Check sheet for the modelled part. Datum: model origin and axes. Units: mm. Face numbers are marked on the shaded views. A direction names the side the tool comes from. Give positions to 0.01 mm unless a question says otherwise; leave off trailing zeros. Write each loop counter-clockwise with the first axis right and the second up, starting at its lowest first coordinate (ties: lowest second). Pieces come first, ordered by that corner, then holes. Notation, with made-up numbers: (-20, 89) -> (4, 89) arc R20 cw to (4, 107) -> close; hole circle Ø10 at (-5, 18). An arc over 180 degrees is marked (long way). Write each question's results on one line, items separated by ' | '. Start each with the question number.
```python
from build123d import *

# Parameters (mm, degrees)
CYLINDER051_R             = 1.6
CYLINDER051_DEPTH         = 28
CYLINDER051_ROLL_ANGLE    = 90
CYLINDER050_R             = 1.6
CYLINDER050_DEPTH         = 28
CYLINDER050_ROLL_ANGLE    = 90
CYLINDER049_R             = 1.6
CYLINDER049_DEPTH         = 28
CYLINDER049_ROLL_ANGLE    = 90
CYLINDER048_R             = 1.6
CYLINDER048_DEPTH         = 28
CYLINDER048_ROLL_ANGLE    = 90
CYLINDER044_R             = 1.6
CYLINDER044_DEPTH         = 28
CYLINDER044_ROLL_ANGLE    = 90
CYLINDER043_R             = 1.6
CYLINDER043_DEPTH         = 28
CYLINDER043_ROLL_ANGLE    = 90
CYLINDER042_R             = 1.6
CYLINDER042_DEPTH         = 28
CYLINDER042_ROLL_ANGLE    = 90
CYLINDER041_R             = 1.6
CYLINDER041_DEPTH         = 28
CYLINDER041_ROLL_ANGLE    = 90
CYLINDER047_R             = 0.85
CYLINDER047_DEPTH         = 10
CYLINDER046_R             = 0.85
CYLINDER046_DEPTH         = 10
FUSION078_PLACEMENT_ANGLE = 90
BOX025_W                  = 22
BOX025_H                  = 4
BOX025_DEPTH              = 5
CYLINDER045_R             = 3.25
CYLINDER045_DEPTH         = 10
CYLINDER045_PITCH_ANGLE   = 90
BOX024_W                  = 55
BOX024_H                  = 31
BOX024_DEPTH              = 13
BOX021_W                  = 61
BOX021_H                  = 34
BOX021_DEPTH              = 13
BOX023_W                  = 12
BOX023_H                  = 3
BOX023_DEPTH              = 13
BOX022_W                  = 12
BOX022_H                  = 3
BOX022_DEPTH              = 13


with BuildPart() as cylinder067:
    # Cylinder051 → Cylinder051 (new body)
    with BuildSketch(Plane.XY):
        Circle(CYLINDER051_R)
    extrude(amount=CYLINDER051_DEPTH)


with BuildPart() as cylinder067_1:
    # Cylinder051 roll: moved
    add(cylinder067.part.rotate(Axis((0, 0, 0), (1, 0, 0)), CYLINDER051_ROLL_ANGLE))


with BuildPart() as cylinder067_2:
    # Cylinder051 placement: moved
    add(cylinder067_1.part.moved(Location((-23, 20, 36))))


with BuildPart() as fusion085:
    # Cylinder050 → Cylinder050 (new body)
    with BuildSketch(Plane.XY):
        Circle(CYLINDER050_R)
    extrude(amount=CYLINDER050_DEPTH)


with BuildPart() as fusion085_1:
    # Cylinder050 roll: moved
    add(fusion085.part.rotate(Axis((0, 0, 0), (1, 0, 0)), CYLINDER050_ROLL_ANGLE))


with BuildPart() as fusion085_2:
    # Cylinder050 placement: moved
    add(fusion085_1.part.moved(Location((-23, 20, 29))))

    # Fusion085: union Cylinder067
    add(cylinder067_2.part)


with BuildPart() as fusion085_3:
    # Fusion085 placement: moved
    add(fusion085_2.part.moved(Location((-1, 0, 0))))


with BuildPart() as cylinder063:
    # Cylinder049 → Cylinder049 (new body)
    with BuildSketch(Plane.XY):
        Circle(CYLINDER049_R)
    extrude(amount=CYLINDER049_DEPTH)


with BuildPart() as cylinder063_1:
    # Cylinder049 roll: moved
    add(cylinder063.part.rotate(Axis((0, 0, 0), (1, 0, 0)), CYLINDER049_ROLL_ANGLE))


with BuildPart() as cylinder063_2:
    # Cylinder049 placement: moved
    add(cylinder063_1.part.moved(Location((-23, 20, 36))))


with BuildPart() as fusion084:
    # Cylinder048 → Cylinder048 (new body)
    with BuildSketch(Plane.XY):
        Circle(CYLINDER048_R)
    extrude(amount=CYLINDER048_DEPTH)


with BuildPart() as fusion084_1:
    # Cylinder048 roll: moved
    add(fusion084.part.rotate(Axis((0, 0, 0), (1, 0, 0)), CYLINDER048_ROLL_ANGLE))


with BuildPart() as fusion084_2:
    # Cylinder048 placement: moved
    add(fusion084_1.part.moved(Location((-23, 20, 29))))

    # Fusion084: union Cylinder063
    add(cylinder063_2.part)


with BuildPart() as fusion084_3:
    # Fusion084 placement: moved
    add(fusion084_2.part.moved(Location((1, 0, 0))))


with BuildPart() as cylinder054:
    # Cylinder044 → Cylinder044 (new body)
    with BuildSketch(Plane.XY):
        Circle(CYLINDER044_R)
    extrude(amount=CYLINDER044_DEPTH)


with BuildPart() as cylinder054_1:
    # Cylinder044 roll: moved
    add(cylinder054.part.rotate(Axis((0, 0, 0), (1, 0, 0)), CYLINDER044_ROLL_ANGLE))


with BuildPart() as cylinder054_2:
    # Cylinder044 placement: moved
    add(cylinder054_1.part.moved(Location((-23, 20, 36))))


with BuildPart() as fusion080:
    # Cylinder043 → Cylinder043 (new body)
    with BuildSketch(Plane.XY):
        Circle(CYLINDER043_R)
    extrude(amount=CYLINDER043_DEPTH)


with BuildPart() as fusion080_1:
    # Cylinder043 roll: moved
    add(fusion080.part.rotate(Axis((0, 0, 0), (1, 0, 0)), CYLINDER043_ROLL_ANGLE))


with BuildPart() as fusion080_2:
    # Cylinder043 placement: moved
    add(fusion080_1.part.moved(Location((-23, 20, 29))))

    # Fusion080: union Cylinder054
    add(cylinder054_2.part)


with BuildPart() as cylinder052:
    # Cylinder042 → Cylinder042 (new body)
    with BuildSketch(Plane.XY):
        Circle(CYLINDER042_R)
    extrude(amount=CYLINDER042_DEPTH)


with BuildPart() as cylinder052_1:
    # Cylinder042 roll: moved
    add(cylinder052.part.rotate(Axis((0, 0, 0), (1, 0, 0)), CYLINDER042_ROLL_ANGLE))


with BuildPart() as cylinder052_2:
    # Cylinder042 placement: moved
    add(cylinder052_1.part.moved(Location((54, 20, 36))))


with BuildPart() as fusion081:
    # Cylinder041 → Cylinder041 (new body)
    with BuildSketch(Plane.XY):
        Circle(CYLINDER041_R)
    extrude(amount=CYLINDER041_DEPTH)


with BuildPart() as fusion081_1:
    # Cylinder041 roll: moved
    add(fusion081.part.rotate(Axis((0, 0, 0), (1, 0, 0)), CYLINDER041_ROLL_ANGLE))


with BuildPart() as fusion081_2:
    # Cylinder041 placement: moved
    add(fusion081_1.part.moved(Location((54, 20, 29))))

    # Fusion081: union Cylinder052
    add(cylinder052_2.part)


with BuildPart() as cylinder059:
    # Cylinder047 → Cylinder047 (new body)
    with BuildSketch(Plane(origin=(10.5, -9, 0), x_dir=(1, 0, 0), z_dir=(0, 0, 1))):
        Circle(CYLINDER047_R)
    extrude(amount=CYLINDER047_DEPTH)


with BuildPart() as fusion078:
    # Cylinder046 → Cylinder046 (new body)
    with BuildSketch(Plane(origin=(10.5, 9, 0), x_dir=(1, 0, 0), z_dir=(0, 0, 1))):
        Circle(CYLINDER046_R)
    extrude(amount=CYLINDER046_DEPTH)

    # Fusion078: union Cylinder059
    add(cylinder059.part)


with BuildPart() as fusion078_1:
    # Fusion078 placement: moved
    add(fusion078.part.moved(Location((14.5, -39, 31))).rotate(Axis((14.5, -39, 31), (0, 0, 1)), FUSION078_PLACEMENT_ANGLE))


with BuildPart() as cut039:
    # Box025 → Box025 (new body)
    with BuildSketch(Plane(origin=(3.5, -31, 34), x_dir=(1, 0, 0), z_dir=(0, 0, 1))):
        with Locations((11, 2)):
            Rectangle(BOX025_W, BOX025_H)
    extrude(amount=BOX025_DEPTH)

    # Cut039: cut Fusion078
    add(fusion078_1.part, mode=Mode.SUBTRACT)


with BuildPart() as cylinder055:
    # Cylinder045 → Cylinder045 (new body)
    with BuildSketch(Plane.XY):
        Circle(CYLINDER045_R)
    extrude(amount=CYLINDER045_DEPTH)


with BuildPart() as cylinder055_1:
    # Cylinder045 pitch: moved
    add(cylinder055.part.rotate(Axis((0, 0, 0), (0, 1, 0)), CYLINDER045_PITCH_ANGLE))


with BuildPart() as cylinder055_2:
    # Cylinder045 placement: moved
    add(cylinder055_1.part.moved(Location((36, -17.25, 32.5))))


with BuildPart() as cube023:
    # Box024 → Box024 (new body)
    with BuildSketch(Plane(origin=(-13, -24, 26), x_dir=(1, 0, 0), z_dir=(0, 0, 1))):
        with Locations((27.5, 15.5)):
            Rectangle(BOX024_W, BOX024_H)
    extrude(amount=BOX024_DEPTH)


with BuildPart() as fusion079:
    # Box021 → Box021 (new body)
    with BuildSketch(Plane(origin=(-16, -27, 26), x_dir=(1, 0, 0), z_dir=(0, 0, 1))):
        with Locations((30.5, 17)):
            Rectangle(BOX021_W, BOX021_H)
    extrude(amount=BOX021_DEPTH)

    # Cut037: cut Cube023
    add(cube023.part, mode=Mode.SUBTRACT)

    # Cut038: cut Cylinder055
    add(cylinder055_2.part, mode=Mode.SUBTRACT)

    # Fusion079: union Cut039
    add(cut039.part)


with BuildPart() as fusion082:
    # Box023 → Box023 (new body)
    with BuildSketch(Plane(origin=(-28, 4, 26), x_dir=(1, 0, 0), z_dir=(0, 0, 1))):
        with Locations((6, 1.5)):
            Rectangle(BOX023_W, BOX023_H)
    extrude(amount=BOX023_DEPTH)

    # Fusion082: union Fusion079
    add(fusion079.part)


with BuildPart() as switch_bracket001:
    # Box022 → Box022 (new body)
    with BuildSketch(Plane(origin=(45, 4, 26), x_dir=(1, 0, 0), z_dir=(0, 0, 1))):
        with Locations((6, 1.5)):
            Rectangle(BOX022_W, BOX022_H)
    extrude(amount=BOX022_DEPTH)

    # Fusion083: union Fusion082
    add(fusion082.part)

    # Cut040: cut Fusion081
    add(fusion081_2.part, mode=Mode.SUBTRACT)

    # Cut041: cut Fusion080
    add(fusion080_2.part, mode=Mode.SUBTRACT)

    # Cut042: cut Fusion084
    add(fusion084_3.part, mode=Mode.SUBTRACT)

    # Cut043: cut Fusion085
    add(fusion085_3.part, mode=Mode.SUBTRACT)


solid = switch_bracket001.part
```
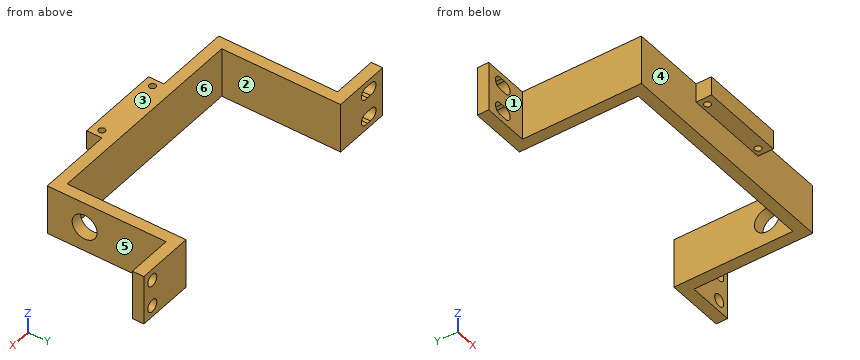
Item 1: Section check B-B on y = -28.5. Record the boundary of the cut face in (x, z), then the cut area to 3 significant figures.
Item 2: Mould release check, pull along X, two halves, no side actions. Record for the marked faces 4, 5 and 6: pulls with the +X half, pulls with the -X half, needs draft (parallel to the pull), parting line crosses it, or undercut.
Item 3: Set-up check for the marked faces 1, 2 and 3: record each of +Z, -Z, +X, -X, +Y, -Y from which the full face is reachable in a straight line by a thin tool's end or side.
Item 4: Section check C-C on z = 32.75. Record the boundary of the cut face in (x, y), then the cut area to 3 significant figures.
Item 5: Thickness scan on probe 1 along Z at (x, y) = (-22, 6.2); probe 2 along X at (y, z) = (6.35, 29); probe 3 along X at (y, z) = (-9, 28.5). Record the ranges inside material, lowest first. Write a range as from..to.
Item 6: Depth check by flat-ended pin: pin 1 Ø1.9 at (x, z) = (-24, 36) entering from +Y; pin 2 Ø6.5 at (x, z) = (11.5, 31.5) entering from +Y; pin 3 Ø5 at (y, z) = (-16, 35.5) entering from -X; pin 4 Ø5 at (y, z) = (-21.5, 35.5) entering from +X. Enter the tip coordinate at first touch or a pass-through.
Item 7: Section check A-A on y = -9. Record the boundary of the cut face in (x, z), then the cut area to 3 significant figures.
Item 8: Section check D-D on x = 2. Record the boundary of the cut face in (y, z), then the cut area to 3 significant figures.
Check sheet entries:
1) outline: (3.5, 34) -> (4.65, 34) -> (4.65, 39) -> (3.5, 39) -> close; (6.35, 34) -> (22.65, 34) -> (22.65, 39) -> (6.35, 39) -> close; (24.35, 34) -> (25.5, 34) -> (25.5, 39) -> (24.35, 39) -> close | area: 93.0 mm^2
2) face 4: needs draft | face 5: pulls with the +X half | face 6: undercut
3) face 1: +Z, -Z, -X, -Y | face 2: +Z, -Z, +Y | face 3: +Z, +X, -X, +Y, -Y
4) outline: (-28, 4) -> (-16, 4) -> (-16, -27) -> (45, -27) -> (45, -20.49) -> (42, -20.49) -> (42, -24) -> (-13, -24) -> (-13, 7) -> (-28, 7) -> close; (42, -14.01) -> (45, -14.01) -> (45, 4) -> (57, 4) -> (57, 7) -> (42, 7) -> close | area: 422 mm^2
5) probe 1: z = 26..27.4, 30.6..34.4, 37.6..39 | probe 2: x = -28..-25.6, -20.4..-13, 42..52.4, 55.6..57 | probe 3: x = -16..-13, 42..45
6) pin 1: passes through | pin 2: stops at y = -24 | pin 3: stops at x = -16 | pin 4: stops at x = 45
7) outline: (-16, 26) -> (-13, 26) -> (-13, 39) -> (-16, 39) -> close; (42, 26) -> (45, 26) -> (45, 39) -> (42, 39) -> close | area: 78.0 mm^2
8) outline: (-27, 26) -> (-24, 26) -> (-24, 39) -> (-27, 39) -> close | area: 39.0 mm^2
